Read the model definition and answer for the solid it produces. Units are mm, in the model's axes. A direction names the side the tool comes from. Round coordinates to 2 decimals unless told otherwise and drop trailing zeros. Loops run counter-clockwise (first coordinate to the right, second up) from the corner with the lowest first, then second, coordinate; pieces in that order, holes last. Notation, with made-up numbers: M 2.5,-0.75 L 38.5,-0.75 A20 cw 38.5,27.25 Z; hole C -18.5,-22 d8. An arc over 180 degrees is marked long. Write each question's results on one line, items separated by ' | '.
from build123d import *

# Parameters (mm, degrees)
BOSS_EXTRUDE1_DEPTH = 25
SKETCH2_R           = 1.75
CUT_EXTRUDE1_DEPTH  = 25
FILLET1_R           = 2
SKETCH4_R           = 2.55
CUT_EXTRUDE2_DEPTH  = 25


with BuildPart() as part:
    # Sketch1 → Boss-Extrude1 (new body)
    with BuildSketch(Plane.XY):
        Polygon((0, 30), (0, 0), (45, 0), (45, 5), (5, 5), (5, 30), align=None)
    extrude(amount=BOSS_EXTRUDE1_DEPTH)

    # Sketch2 → Cut-Extrude1 (cut)
    with BuildSketch(Plane(origin=(5, 0, 0), x_dir=(0, 0, -1), z_dir=(1, 0, 0))):
        with Locations((-12.5, 17.5)):
            Circle(SKETCH2_R)
    extrude(amount=-CUT_EXTRUDE1_DEPTH, mode=Mode.SUBTRACT)

    # Fillet1
    fillet1_edges = [part.edges().sort_by_distance(p)[0] for p in [
        (5, 5, 12.5),
    ]]
    fillet(fillet1_edges, radius=FILLET1_R)

    # Sketch4 → Cut-Extrude2 (cut)
    with BuildSketch(Plane(origin=(0, 5, 0), x_dir=(1, 0, 0), z_dir=(0, 1, 0))):
        with Locations((35, -12.5)):
            Circle(SKETCH4_R)
        with Locations((15, -12.5)):
            Circle(SKETCH4_R)
    extrude(amount=-CUT_EXTRUDE2_DEPTH, mode=Mode.SUBTRACT)


solid = part.part
Item 1: The part is cut by section B-B (y = 17.5). Determine the outline of the cut face in (x, z), plus the area to 4 significant figures.
Outcome:
outline: M 0,0 L 5,0 L 5,10.75 L 0,10.75 Z; M 0,14.25 L 5,14.25 L 5,25 L 0,25 Z | area: 107.5 mm2
Item 2: For faces 1 (the face through (32.452, 2.535, 12.388)), 2 (the face through (5, 21, 12)), determine the directions among +Z, -Z, +X, -X, +Y, -Y from which every point of the face is accessible in a straight line to the end or side of a thin tool.
Outcome:
face 1: +Y, -Y | face 2: +Z, -Z, +X, +Y
Item 3: The mould has two halves that part along X. Classify faces 3 (the face through (5.57, 5.6, 12.68)), 4 (the face through (12.976, 2.535, 14.052)), 5 (the face through (22, 0, 12)): pulls with the +X half, pulls with the -X half, needs draft (parallel to the pull), parting line crosses it, or undercut.
Outcome:
face 3: pulls with the +X half | face 4: undercut | face 5: needs draft
Item 4: Flat-ended cylindrical pins translate along their axes: pin 1 (5.5 mm diameter, centred on y = 17.5, z = 12.5, fed in from -X); pin 2 (6 mm diameter, centred on x = 39.5, z = 17.5, fed in from +Y); pin 3 (3 mm diameter, centred on y = 20.5, z = 10.5, fed in from +X). Find the tip coordinate at first contact, or state that the pin passes through.
Outcome:
pin 1: stops at x = 0 | pin 2: stops at y = 5 | pin 3: stops at x = 5
Item 5: Straight lines are drawn through the part: line 1 (X direction, y = 1.7, z = 12.5); line 2 (Z direction, x = 35, y = 4.05); line 3 (Y direction, x = 2.1, z = 12.5). For each, find the intervals that lie inside material, in ascending order.
Outcome:
line 1: x = 0 to 12.45, 17.55 to 32.45, 37.55 to 45 | line 2: z = 0 to 9.95, 15.05 to 25 | line 3: y = 0 to 15.75, 19.25 to 30
Item 6: The part is cut by section C-C (x = 35). Determine the outline of the cut face in (y, z), plus the area to 3 significant figures.
Outcome:
outline: M 0,0 L 5,0 L 5,9.95 L 0,9.95 Z; M 0,15.05 L 5,15.05 L 5,25 L 0,25 Z | area: 99.5 mm2
Item 7: The part is cut by section A-A (z = 12.5). Determine the outline of the cut face in (x, y), plus the area to 3 significant figures.
Outcome:
outline: M 0,0 L 12.45,0 L 12.45,5 L 7,5 A2 cw 5,7 L 5,15.75 L 0,15.75 Z; M 0,19.25 L 5,19.25 L 5,30 L 0,30 Z; M 17.55,0 L 32.45,0 L 32.45,5 L 17.55,5 Z; M 37.55,0 L 45,0 L 45,5 L 37.55,5 Z | area: 282 mm2
Item 8: The part is cut by section D-D (y = 3). Determine the outline of the cut face in (x, z).
Outcome:
outline: M 0,0 L 45,0 L 45,25 L 0,25 Z; hole C 15,12.5 d5.1; hole C 35,12.5 d5.1
